```python
from build123d import *

# Parameters (mm, degrees)
SKETCH1_W           = 152.4
SKETCH1_H           = 25.4
BOSS_EXTRUDE1_DEPTH = 1.5875
SKETCH2_W           = 3.175
SKETCH2_H           = 3.175
BOSS_EXTRUDE2_DEPTH = 152.4


with BuildPart() as part:
    # Sketch1 → Boss-Extrude1 (new body)
    with BuildSketch(Plane.XY):
        with Locations((-15.173816053, 41.697804783)):
            Rectangle(SKETCH1_W, SKETCH1_H)
    extrude(amount=BOSS_EXTRUDE1_DEPTH)

    # Sketch2 → Boss-Extrude2 (add)
    with BuildSketch(Plane.ZY.offset(91.373816053)):
        with Locations((0.79375, 27.410304783)):
            Rectangle(SKETCH2_W, SKETCH2_H)
    extrude(amount=-BOSS_EXTRUDE2_DEPTH)


solid = part.part
```
Input: part model. Units: mm. Frame: model coordinates. A direction names the side the tool comes from. Give positions to 0.01 mm unless a question says otherwise; leave off trailing zeros. Loops run counter-clockwise (first coordinate to the right, second up) from the corner with the lowest first, then second, coordinate; pieces in that order, holes last.
1) Mould query, pull axis X, two halves, no side actions, for faces 4 (the flat face through (-91.374, 40, 1)), 5 (the flat face through (-16, 27, 2.381)), 6 (the flat face through (61.026, 40, 1)). Classes: released by +X, released by -X, zero draft, split by the parting line, or undercut.
A:
face 4: released by -X
face 5: zero draft
face 6: released by +X
2) Contact query for flat-ended pins moving along their axis: pin 1 (7.5 mm diameter, centred on x = 14, y = 45.5, fed in from +Z); pin 2 (5 mm diameter, centred on x = -21, y = 37.5, fed in from -Z). Output: stop coordinate, or through.
A:
pin 1: stops at z = 1.59
pin 2: stops at z = 0
3) Section query A-A on x = -7. Return the cut outline in (y, z).
A:
outline: (25.82, -0.79) - (29, -0.79) - (29, 0) - (54.4, 0) - (54.4, 1.59) - (29, 1.59) - (29, 2.38) - (25.82, 2.38) - close
4) Section query B-B on y = 42.25. Return the cut outline in (x, z), and give its area (3 significant figures).
A:
outline: (-91.37, 0) - (61.03, 0) - (61.03, 1.59) - (-91.37, 1.59) - close
area: 242 mm2
5) Reachability of faces 1 (the flat face through (-16, 27, -0.794)), 2 (the flat face through (-16, 42, 0)), 3 (the flat face through (-16, 42, 1.588)) from +Z, -Z, +X, -X, +Y, -Y: full face, straight path, thin tool, end or side. Return the list, or none.
A:
face 1: -Z, +X, -X, +Y, -Y
face 2: -Z, +X, -X, +Y
face 3: +Z, +X, -X, +Y
6) Line query: L1, parallel to Z at x = 1, y = 45.5; L2, parallel to Y at x = 43.5, z = -0.4. Output: solid intervals per line, ascending.
A:
L1: z = 0 to 1.59
L2: y = 25.82 to 29
